Here's how the part is built. I have some questions about the finished solid (model axes, mm). Face numbers are marked on the shaded views. A direction names the side the tool comes from. Coordinates: 2 decimals unless noted, no trailing zeros. Write each loop counter-clockwise with the first axis right and the second up, starting at its lowest first coordinate (ties: lowest second). Pieces come first, ordered by that corner, then holes. Notation, with made-up numbers: M -15,83.25 L 39,83.25 A24 cw 39,103.25 Z; hole C 71,45 d5. An arc over 180 degrees is marked long. Use a Markdown table: item, result.
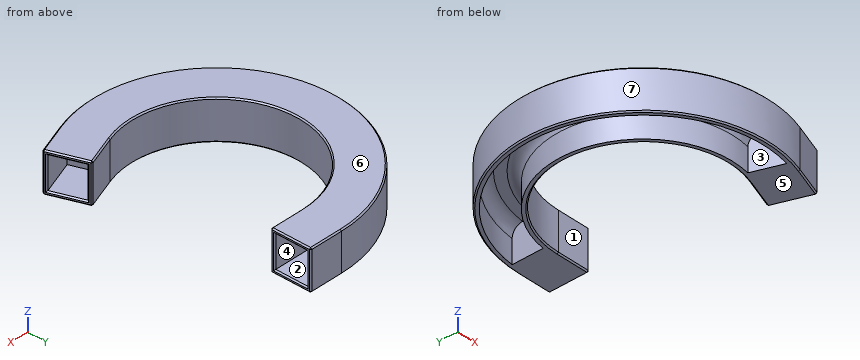
```python
from build123d import *

# Parameters (mm, degrees)
F1_DEPTH  = 19.2
F2_DEPTH  = 16
F3_DEPTH  = 16
F4_W      = 15.4
F4_H      = 15.4
F5_DEPTH  = 18
F6_W      = 15.4
F6_H      = 15.4
F7_DEPTH  = 18
F8_SIZE   = 0.6
F10_DEPTH = 16.2
F11_R     = 5


with BuildPart() as f1:
    # F0 (on Top) → F1 (new body)
    with BuildSketch(Plane.XY):
        with BuildLine():
            Line((0, 40.8), (0, 60))
            ThreePointArc((0, 60), (-59.0884651807, -10.41889066), (20.5212085995, -56.3815572472))
            Line((20.5212085995, -56.3815572472), (13.9544218477, -38.3394589281))
            ThreePointArc((13.9544218477, -38.3394589281), (-40.1801563229, -7.0848456488), (0, 40.8))
        make_face()
    extrude(amount=F1_DEPTH)

    # F2 (add): a face of the model
    f2_faces = [f1.faces().sort_by_distance(p)[0] for p in [
        (0, 50.4, 9.6),
    ]]
    extrude(f2_faces, amount=F2_DEPTH)

    # F3 (add): a face of the model
    f3_faces = [f1.faces().sort_by_distance(p)[0] for p in [
        (17.2378152236, -47.3605080876, 9.6),
    ]]
    extrude(f3_faces, amount=F3_DEPTH)

    # F4 (on face) → F5 (cut)
    with BuildSketch(Plane.YZ.offset(16)):
        with Locations((50.4, 9.6)):
            Rectangle(F4_W, F4_H)
    extrude(amount=-F5_DEPTH, mode=Mode.SUBTRACT)

    # F6 (on face) → F7 (cut)
    with BuildSketch(Plane(origin=(15.0350819326, 5.4723222932, 0), x_dir=(-0.3420201433, 0.9396926208, 0), z_dir=(0.9396926208, 0.3420201433, 0))):
        with Locations((-50.4, 9.6)):
            Rectangle(F6_W, F6_H)
    extrude(amount=-F7_DEPTH, mode=Mode.SUBTRACT)

    # F8
    f8_edges = [f1.edges().sort_by_distance(p)[0] for p in [
        (-40.180156, -7.084846, 19.2),
        (-59.088465, -10.418891, 19.2),
        (-40.180156, -7.084846, 0),
        (-59.088465, -10.418891, 0),
        (16, 40.8, 9.6),
        (16, 50.4, 0),
        (16, 50.4, 19.2),
        (16, 60, 9.6),
        (16, 50.4, 17.3),
        (16, 58.1, 9.6),
        (16, 50.4, 1.9),
        (16, 42.7, 9.6),
        (35.556291, -50.909235, 9.6),
        (32.272897, -41.888186, 0),
        (32.272897, -41.888186, 19.2),
        (28.989504, -32.867137, 9.6),
        (32.272897, -41.888186, 17.3),
        (29.639342, -34.652553, 9.6),
        (32.272897, -41.888186, 1.9),
        (34.906452, -49.123819, 9.6),
    ]]
    chamfer(f8_edges, length=F8_SIZE)

    # F9 (on face) → F10 (cut)
    with BuildSketch(Plane(origin=(0, 0, 0), x_dir=(1, 0, 0), z_dir=(0, 0, -1))):
        with BuildLine():
            Line((8.9248354623, 42.063610306), (14.023808605, 56.0729238779))
            ThreePointArc((14.023808605, 56.0729238779), (-56.9218881241, 10.0368646691), (-6, -57.4877378229))
            Line((-6, -57.4877378229), (-6, -42.5793377121))
            ThreePointArc((-6, -42.5793377121), (-42.3467333795, 7.4668716397), (8.9248354623, 42.063610306))
        make_face()
    extrude(amount=-F10_DEPTH, mode=Mode.SUBTRACT)

    # F11
    f11_edges = [f1.edges().sort_by_distance(p)[0] for p in [
        (-56.921888, -10.036865, 16.2),
        (-42.346733, -7.466872, 16.2),
    ]]
    fillet(f11_edges, radius=F11_R)


solid = f1.part
```
1. Which directions (+Z, -Z, +X, -X, +Y, -Y) give clear straight access to the entire face, cutting with the end or side of a thin tool? Please do the marked faces 1, 2 and 3.
Answers follow:
| item | result |
|---|---|
| face 1 | +Z, -Z, +X |
| face 2 | +X |
| face 3 | -Z |
2. I need wall thicknesses on probe 1 along Y at (x, z) = (0, 6.25); probe 2 along X at (y, z) = (0, 11.75); probe 3 along Y at (x, z) = (-33, 1). Which ranges of each line are inside material? Lowest first, please.
Answers follow:
| item | result |
|---|---|
| probe 1 | y = -60 to -57.8, -43 to -40.8, 40.8 to 42.7, 58.1 to 60 |
| probe 2 | x = -60 to -57.77, -43.03 to -40.8 |
| probe 3 | y = -50.11 to -47.45, -27.57 to -23.99, 23.99 to 27.57, 47.45 to 50.11 |
3. We'd pull the mould along Z, two halves only. Please class the marked faces 4, 5, 6 and 7: +Z half, -Z half, draft (parallel to the pull), parting line (faces both ways), or undercut.
Answers follow:
| item | result |
|---|---|
| face 4 | undercut |
| face 5 | -Z half |
| face 6 | +Z half |
| face 7 | draft |
4. Suppose I cut it at A-A on z = 9.5. Write out the boundary of the cut face in (x, y), and give its area (3 significant figures).
Answers follow:
| item | result |
|---|---|
| outline | M -2,42.7 L -2,58.1 L 15.4,58.1 L 16,58.7 L 16,59.4 L 15.4,60 L 0,60 A60 ccw long 20.52,-56.38 L 34.99,-51.11 L 35.35,-50.35 L 35.11,-49.69 L 34.34,-49.33 L 17.99,-55.28 L 12.72,-40.81 L 29.08,-34.86 L 29.43,-34.09 L 29.19,-33.43 L 28.43,-33.07 L 13.95,-38.34 A40.8 cw long 0,40.8 L 15.4,40.8 L 16,41.4 L 16,42.1 L 15.4,42.7 Z; hole M -6,42.58 L -6,57.49 A57.8 ccw long 14.02,-56.07 L 8.92,-42.06 A43 cw long Z |
| area | 1,010 mm2 |
5. Will these pins go through, and if not, where does the flat tip stop? pin 1 Ø7.5 at (y, z) = (49, 9.5) entering from +X; pin 2 Ø4 at (x, z) = (23.5, 17) entering from -Y; pin 3 Ø10 at (x, z) = (-22, 4.5) entering from +Y; pin 4 Ø3 at (x, y) = (-34.5, 15.5) entering from -Z.
Answers follow:
| item | result |
|---|---|
| pin 1 | stops at x = -2 |
| pin 2 | stops at y = -56.03 |
| pin 3 | stops at y = 57.54 |
| pin 4 | passes through |
